Build history of the part. All positions in model axes, mm. Round coordinates to 2 decimals unless told otherwise and drop trailing zeros. Use a Markdown table: item, result. Add a question column.
Item 1: Two-plate mould, pull along Y, no slides. Class faces 1 (the face through (-51.42, 73.17, 3.04)), 2 (the face through (7.97, 28.16, 2.96)), 3 (the face through (67.724, -45.971, 3.042)), 4 (the face through (7, 15, 6)): released by +Y, released by -Y, zero draft, split by the parting line, or undercut.
Item 2: Slice it at A-A, the plane z = 2.55. State how many separate pieces and enclosed holes the cut face has, plus the area to 3 significant figures.
Item 3: Probe L1, parallel to Y at x = 44, z = 2.7; L2, parallel to Y at x = -42.5, z = 1.5; L3, parallel to X at y = 65, z = 5.35. List the from-to ranges inside material, lowest first.
Item 4: Pin check, flat tips, straight feed: pin 1 (4.5 mm diameter, centred on x = -41.77, y = 63.68, fed in from +Z); pin 2 (2.5 mm diameter, centred on x = 33.23, y = -11.32, fed in from -Z). Stop position of each tip, or through.
from build123d import *

# Parameters (mm, degrees)
F0_W     = 125
F0_H     = 125
F0_R     = 2
F1_DEPTH = 6
F2_R     = 10


with BuildPart() as f1:
    # F0 (on Top) → F1 (new body)
    with BuildSketch(Plane.XY):
        with Locations((8.230951, 13.677106)):
            Rectangle(F0_W, F0_H)
        with Locations((-41.769049, -36.322894)):
            Circle(F0_R, mode=Mode.SUBTRACT)
        with Locations((-29.269049, -23.822894)):
            Circle(F0_R, mode=Mode.SUBTRACT)
        with Locations((-16.769049, -11.322894)):
            Circle(F0_R, mode=Mode.SUBTRACT)
        with Locations((58.230951, -36.322894)):
            Circle(F0_R, mode=Mode.SUBTRACT)
        with Locations((45.730951, -23.822894)):
            Circle(F0_R, mode=Mode.SUBTRACT)
        with Locations((33.230951, -11.322894)):
            Circle(F0_R, mode=Mode.SUBTRACT)
        with Locations((8.230951, 1.177106)):
            Circle(F0_R, mode=Mode.SUBTRACT)
        with Locations((-16.769049, 38.677106)):
            Circle(F0_R, mode=Mode.SUBTRACT)
        with Locations((-29.269049, 51.177106)):
            Circle(F0_R, mode=Mode.SUBTRACT)
        with Locations((-41.769049, 63.677106)):
            Circle(F0_R, mode=Mode.SUBTRACT)
        with Locations((8.230951, 26.177108)):
            Circle(F0_R, mode=Mode.SUBTRACT)
        with Locations((33.230951, 38.677106)):
            Circle(F0_R, mode=Mode.SUBTRACT)
        with Locations((45.730951, 51.177106)):
            Circle(F0_R, mode=Mode.SUBTRACT)
        with Locations((58.230951, 63.677106)):
            Circle(F0_R, mode=Mode.SUBTRACT)
    extrude(amount=F1_DEPTH)

    # F2
    f2_edges = [f1.edges().sort_by_distance(p)[0] for p in [
        (-54.269049, 76.177106, 3),
        (-54.269049, -48.822894, 3),
        (70.730951, -48.822894, 3),
        (70.730951, 76.177106, 3),
    ]]
    fillet(f2_edges, radius=F2_R)


solid = f1.part
Check sheet entries:
| question | item | result |
|---|---|---|
| 1 | face 1 | released by +Y |
| 1 | face 2 | undercut |
| 1 | face 3 | released by -Y |
| 1 | face 4 | zero draft |
| 2 | separate pieces | 1 |
| 2 | enclosed holes | 14 |
| 2 | area | 15,400 mm2 |
| 3 | L1 | -48.82 to -24.82, -22.82 to 50.18, 52.18 to 76.18 |
| 3 | L2 | -48.82 to -38.18, -34.46 to 61.82, 65.54 to 76.18 |
| 3 | L3 | -54.27 to -43.27, -40.27 to 56.73, 59.73 to 70.73 |
| 4 | pin 1 | z = 6 |
| 4 | pin 2 | through |
